Build history of the part. All positions in model axes, mm. A direction names the side the tool comes from. Give positions to 0.01 mm unless a question says otherwise; leave off trailing zeros. Order: outer loops, then holes, each group sorted by start corner. A loop starts at its lowest first (then second) coordinate and runs counter-clockwise, first axis right, second up. Notation, with made-up numbers: (62.5, 55.25) -> (107.5, 55.25) arc R24 cw to (107.5, 70.25) -> close; hole circle Ø6 at (20, -18.75). An arc over 180 degrees is marked (long way). One line per question, with ' | ' between items. Start each with the question number.
(1) Pin check, flat tips, straight feed: pin 1 Ø10 at (x, z) = (110, -23.5) entering from +Y; pin 2 Ø8 at (x, z) = (49, -44) entering from +Y; pin 3 Ø14.5 at (y, z) = (34, -61) entering from +X; pin 4 Ø4 at (y, z) = (19.5, -47.5) entering from -X. Stop position of each tip, or through.
(2) Cut at C-C (x = 63.5). Give the cut face in (y, z).
(3) Cut at A-A (y = 19.5). Give the cut face in (x, z).
(4) Which spindle directions (+Z, -Z, +X, -X, +Y, -Y) get a long thin tool onto all of the face, cutting with end or side? Do faces 4 (the face through (52, 2, -49)), 5 (the face through (46, 1, 0)), 6 (the face through (0, 26, -49)). Say none if no direction does.
(5) Pull direction X, two halves, no side cores. Call faces 1 (the face through (-25, 50, -49)), 2 (the face through (120.015, 10.42, -49.3)), 3 (the face through (120.979, 8.555, -49.3)): +X half, -X half, draft (parallel to the pull), parting line (faces both ways), or undercut.
(6) Cut at B-B (z = -32.5). Give the cut face in (x, y).
(7) Cut at D-D (y = 27). Give the cut face in (x, z), then the cut area to 3 significant figures.
(8) Drill centre lines: L1, parallel to Y at x = -6, z = -83; L2, parallel to X at y = 6.5, z = -15.5; L3, parallel to X at y = 11, z = -6. Where is each one in solid material? Low to high. Write a range as from..to.
from build123d import *

# Parameters (mm, degrees)
SM_BASE_FLANGE_1_DEPTH = 100


# Sheet-metal steps are written as plain solids
with BuildPart() as part:
    # Sketch 1 → 基体-法兰1 (new body)
    with BuildSketch(Plane.XY):
        with BuildLine():
            Line((-50, 50), (-0.1, 50))
            ThreePointArc((-0.1, 50), (-0.029289322, 49.970710678), (0, 49.9))
            Line((0, 49.9), (0, 2.1))
            ThreePointArc((0, 2.1), (0.61507576, 0.61507576), (2.1, 0))
            Line((2.1, 0), (100, 0))
            ThreePointArc((100, 0), (121.213203436, 8.786796564), (130, 30))
            Line((130, 30), (128, 30))
            ThreePointArc((128, 30), (119.798989873, 10.201010127), (100, 2))
            Line((100, 2), (2.1, 2))
            ThreePointArc((2.1, 2), (2.029289322, 2.029289322), (2, 2.1))
            Line((2, 2.1), (2, 49.9))
            ThreePointArc((2, 49.9), (1.384924241, 51.38492424), (-0.1, 52))
            Line((-0.1, 52), (-50, 52))
            Line((-50, 52), (-50, 50))
        make_face()
    extrude(amount=-SM_BASE_FLANGE_1_DEPTH)


solid = part.part
Result set:
1) pin 1: stops at y = 6.36 | pin 2: stops at y = 2 | pin 3: stops at x = 130 | pin 4: stops at x = 0
2) outline: (0, -100) -> (2, -100) -> (2, 0) -> (0, 0) -> close
3) outline: (0, -100) -> (2, -100) -> (2, 0) -> (0, 0) -> close; (125.96, -100) -> (128.1, -100) -> (128.1, 0) -> (125.96, 0) -> close
4) face 4: +Z, -Z, +Y | face 5: +Z, +X, -X, +Y, -Y | face 6: +Z, -Z, -X, -Y
5) face 1: draft | face 2: undercut | face 3: +X half
6) outline: (-50, 50) -> (-0.1, 50) arc R0.1 cw to (0, 49.9) -> (0, 2.1) arc R2.1 ccw to (2.1, 0) -> (100, 0) arc R30 ccw to (130, 30) -> (128, 30) arc R28 cw to (100, 2) -> (2.1, 2) arc R0.1 cw to (2, 2.1) -> (2, 49.9) arc R2.1 ccw to (-0.1, 52) -> (-50, 52) -> close
7) outline: (0, -100) -> (2, -100) -> (2, 0) -> (0, 0) -> close; (127.84, -100) -> (129.85, -100) -> (129.85, 0) -> (127.84, 0) -> close | area: 401 mm2
8) L1: y = 50..52 | L2: x = 0..2, 115.22..118.65 | L3: x = 0..2, 120.57..123.22
